from build123d import *

# Parameters (mm, degrees)
SKETCH1_W                                = 56
SKETCH1_H                                = 56
BOSS_EXTRUDE1_DEPTH                      = 44
SKETCH2_W                                = 56.5
SKETCH2_H                                = 56.5
SKETCH2_R                                = 2.3
BOSS_EXTRUDE2_DEPTH                      = 5
SKETCH3_R                                = 19.851731711
SKETCH3_R_2                              = 16.528882373
CUT_EXTRUDE1_DEPTH                       = 3
SKETCH4_R                                = 3.25
BOSS_EXTRUDE3_DEPTH                      = 20
CUT_EXTRUDE2_DEPTH                       = 44
MIRROR1_AT_THE_SECOND_PLANE_COPY_1_DEPTH = 44
FILLET3_R                                = 1
FILLET2_R                                = 5


with BuildPart() as part:
    # Sketch1 → Boss-Extrude1 (new body)
    with BuildSketch(Plane(origin=(0, 0, 0), x_dir=(1, 0, 0), z_dir=(0, 1, 0))):
        Rectangle(SKETCH1_W, SKETCH1_H)
    extrude(amount=BOSS_EXTRUDE1_DEPTH)

    # Sketch2 → Boss-Extrude2 (add)
    with BuildSketch(Plane(origin=(0, 44, 0), x_dir=(1, 0, 0), z_dir=(0, 1, 0))):
        Rectangle(SKETCH2_W, SKETCH2_H)
        with Locations((-24, 24)):
            Circle(SKETCH2_R, mode=Mode.SUBTRACT)
        with Locations((24, 24)):
            Circle(SKETCH2_R, mode=Mode.SUBTRACT)
        with Locations((-24, -24)):
            Circle(SKETCH2_R, mode=Mode.SUBTRACT)
        with Locations((24, -24)):
            Circle(SKETCH2_R, mode=Mode.SUBTRACT)
    extrude(amount=BOSS_EXTRUDE2_DEPTH)

    # Sketch3 → Cut-Extrude1 (cut)
    with BuildSketch(Plane(origin=(0, 49, 0), x_dir=(1, 0, 0), z_dir=(0, 1, 0))):
        Circle(SKETCH3_R)
        Circle(SKETCH3_R_2, mode=Mode.SUBTRACT)
    extrude(amount=-CUT_EXTRUDE1_DEPTH, mode=Mode.SUBTRACT)

    # Sketch4 → Boss-Extrude3 (add)
    with BuildSketch(Plane(origin=(0, 49, 0), x_dir=(1, 0, 0), z_dir=(0, 1, 0))):
        Circle(SKETCH4_R)
    extrude(amount=BOSS_EXTRUDE3_DEPTH)

    # Sketch5 → Cut-Extrude2 (cut)
    with BuildSketch(Plane.XZ):
        with BuildLine():
            Line((-28, 18), (-28, 28))
            Line((-28, 28), (-18, 28))
            ThreePointArc((-18, 28), (-20.83143897, 20.83143897), (-28, 18))
        make_face()
    cut_extrude2 = extrude(amount=-CUT_EXTRUDE2_DEPTH, mode=Mode.SUBTRACT)

    # Mirror1: Cut-Extrude2 across plane
    add(cut_extrude2.mirror(Plane(origin=(0, 0, 0), x_dir=(0, 0, 1), z_dir=(1, 0, 0))), mode=Mode.SUBTRACT)

    # Mirror1 at the second plane: Cut-Extrude2 across plane
    add(cut_extrude2.mirror(Plane.XY), mode=Mode.SUBTRACT)

    # Mirror1 at the second plane copy 1 sketc → Mirror1 at the second plane copy 1 (cut)
    with BuildSketch(Plane(origin=(0, 0, 0), x_dir=(-1, 0, 0), z_dir=(0, -1, 0))):
        with BuildLine():
            Line((-28, 18), (-28, 28))
            Line((-28, 28), (-18, 28))
            ThreePointArc((-18, 28), (-20.83143897, 20.83143897), (-28, 18))
        make_face()
    extrude(amount=-MIRROR1_AT_THE_SECOND_PLANE_COPY_1_DEPTH, mode=Mode.SUBTRACT)

    # Fillet3
    fillet3_edges = [part.edges().sort_by_distance(p)[0] for p in [
        (-18, 22, 28),
        (-28, 22, 18),
        (-28, 22, -18),
        (-18, 22, -28),
        (28, 22, 18),
        (18, 22, 28),
        (18, 22, -28),
        (28, 22, -18),
    ]]
    fillet(fillet3_edges, radius=FILLET3_R)

    # Fillet2
    fillet2_edges = [part.edges().sort_by_distance(p)[0] for p in [
        (28.25, 46.5, 28.25),
        (28.25, 46.5, -28.25),
        (-28.25, 46.5, -28.25),
        (-28.25, 46.5, 28.25),
    ]]
    fillet(fillet2_edges, radius=FILLET2_R)


solid = part.part
Can you work these out from the model? Positions are in its coordinate system, mm. A direction names the side the tool comes from. Give positions to 0.01 mm unless a question says otherwise; leave off trailing zeros. Loops run counter-clockwise (first coordinate to the right, second up) from the corner with the lowest first, then second, coordinate; pieces in that order, holes last. Notation, with made-up numbers: (78.5, 89) -> (105.5, 89) arc R22 ccw to (105.5, 96) -> close; hole circle Ø11 at (85, 81.5). An arc over 180 degrees is marked (long way). Return JSON: item names as keys, results as strings.
Q1. I want a section at A-A, the plane y = 16. List the corners of the cut face in (x, z) for me.
Checks:
{"outline": "(-28, -17.02) arc R1 ccw to (-27.06, -18.01) arc R9.69 cw to (-18.01, -27.06) arc R1 ccw to (-17.02, -28) -> (17.02, -28) arc R1 ccw to (18.01, -27.06) arc R9.69 cw to (27.06, -18.01) arc R1 ccw to (28, -17.02) -> (28, 17.02) arc R1 ccw to (27.06, 18.01) arc R9.69 cw to (18.01, 27.06) arc R1 ccw to (17.02, 28) -> (-17.02, 28) arc R1 ccw to (-18.01, 27.06) arc R9.69 cw to (-27.06, 18.01) arc R1 ccw to (-28, 17.02) -> close"}
Q2. We'd pull the mould along Z, two halves only. Please class faces 5 (the face through (18.935, 47.521, -5.963)), 6 (the face through (20.763, 21.692, -20.901)), 7 (the face through (-28.25, 46, 0)): released by +Z, released by -Z, zero draft, split by the parting line, or undercut.
Checks:
{"face 5": "undercut", "face 6": "released by -Z", "face 7": "zero draft"}
Q3. I want a section at B-B, the plane x = 0. List the corners of the cut face in (y, z) for me.
Checks:
{"outline": "(0, -28) -> (44, -28) -> (44, -28.25) -> (49, -28.25) -> (49, -19.85) -> (46, -19.85) -> (46, -16.53) -> (49, -16.53) -> (49, -3.25) -> (69, -3.25) -> (69, 3.25) -> (49, 3.25) -> (49, 16.53) -> (46, 16.53) -> (46, 19.85) -> (49, 19.85) -> (49, 28.25) -> (44, 28.25) -> (44, 28) -> (0, 28) -> close"}
Q4. On a 3-axis mill with a long thin cutter (end or side, diameter ignored), from which of +Z, -Z, +X, -X, +Y, -Y can I reach the whole of each face in a straight line? I mean faces 1 (the face through (20.763, 21.692, 20.901)), 2 (the face through (-13.117, 47.521, 10.058)), 3 (the face through (28, 22, 0)), 4 (the face through (-28, 22, 0)). Say none if no direction works.
Checks:
{"face 1": "+Z, +X, -Y", "face 2": "+Y", "face 3": "+Z, -Z, +X, -Y", "face 4": "+Z, -Z, -X, -Y"}
Q5. I want a section at C-C, the plane z = 15.5. List the corners of the cut face in (x, y) for me, then the cut area to 3 significant figures.
Checks:
{"outline": "(-28.25, 44) -> (-28, 44) -> (-28, 0) -> (28, 0) -> (28, 44) -> (28.25, 44) -> (28.25, 49) -> (12.4, 49) -> (12.4, 46) -> (5.74, 46) -> (5.74, 49) -> (-5.74, 49) -> (-5.74, 46) -> (-12.4, 46) -> (-12.4, 49) -> (-28.25, 49) -> close", "area": "2,710 mm2"}
Q6. For pin 1 Ø6 at (x, z) = (24, 24) entering from +Y; pin 2 Ø10 at (x, y) = (4.5, 20.5) entering from +Z; pin 3 Ø5.5 at (x, z) = (-24, -24) entering from -Y, each with a flat end and sliding along its axis, tell me the tip position at first contact or that it passes through.
Checks:
{"pin 1": "stops at y = 49", "pin 2": "stops at z = 28", "pin 3": "stops at y = 44"}
Q7. I need wall thicknesses on probe 1 along X at (y, z) = (46.9, 0); probe 2 along X at (y, z) = (46.25, -24). Which ranges of each line are inside material? Lowest first, please.
Checks:
{"probe 1": "x = -28.25 to -19.85, -16.53 to 16.53, 19.85 to 28.25", "probe 2": "x = -28.19 to -26.3, -21.7 to 21.7, 26.3 to 28.19"}
